For this review, take the finished solid that the model builds, in its own axes (mm). A direction names the side the tool comes from. Give positions to 0.01 mm unless a question says otherwise; leave off trailing zeros. Loops run counter-clockwise (first coordinate to the right, second up) from the corner with the lowest first, then second, coordinate; pieces in that order, holes last.
```python
from build123d import *

# Parameters (mm, degrees)
F0_W     = 20
F0_H     = 20
F1_DEPTH = 23
F2_W     = 20
F2_H     = 20
F3_DEPTH = 2
F3_TAPER = 30
F6_R     = 2


with BuildPart() as f1:
    # F0 (on Top) → F1 (new body)
    with BuildSketch(Plane.XY):
        Rectangle(F0_W, F0_H)
    extrude(amount=F1_DEPTH)

    # F2 (on face) → F3 (join)
    with BuildSketch(Plane.XY.offset(23)):
        Rectangle(F2_W, F2_H)
    extrude(amount=F3_DEPTH, taper=F3_TAPER)

    # F4 (on Front) → F5 (revolve)
    with BuildSketch(Plane.XZ):
        Polygon((0, -56), (0, 0), (-10, 0), (-7, -8), (-7, -50), (-5, -50), (-5, -56), align=None)
    revolve(axis=Axis((0, 0, -28), (0, 0, -1)))

    # F6
    f6_edges = [f1.edges().sort_by_distance(p)[0] for p in [
        (-10, 10, 11.5),
        (-10, -10, 11.5),
        (10, -10, 11.5),
        (10, 10, 11.5),
    ]]
    fillet(f6_edges, radius=F6_R)


solid = f1.part
```
Q1. For pin 1 Ø1 at (y, z) = (6, -42) entering from +X; pin 2 Ø11 at (x, y) = (-5.5, 7.5) entering from -Z; pin 3 Ø3 at (x, y) = (-4.5, -6.5) entering from -Z; pin 4 Ø1 at (x, z) = (-5.5, -46) entering from -Y, all flat-tipped, find the tip position at first contact; note any pin that passes through.
Answers:
pin 1: stops at x = 4.33
pin 2: stops at z = -56
pin 3: stops at z = -50
pin 4: stops at y = -4.9
Q2. For probe 1 along Z at (x, y) = (-2.75, -6); probe 2 along Z at (x, y) = (7.25, 7.25); probe 3 along X at (y, z) = (5.5, -10), list the stretches that pass through material, from the lowest coordinate up.
Answers:
probe 1: z = -50 to 25
probe 2: z = 0 to 25
probe 3: x = -4.33 to 4.33
Q3. Mouldability with a two-part tool opening along X and no side actions: class faces 1 (the cylindrical face through (-9.43, -9.4, 12.18)), 2 (the cylindrical face through (9.4, -9.43, 12.18)), 3 (the flat face through (2, 5, -50)) as +X half, -X half, draft (parallel to the pull), parting line (faces both ways), or undercut.
Answers:
face 1: -X half
face 2: +X half
face 3: draft
Q4. Consider section A-A on z = -15.5. Give the boundary of the cut face in (x, y), plus the area to 3 significant figures.
Answers:
outline: circle Ø14 at (0, 0)
area: 154 mm2
Q5. Machinability: for faces 4 (the flat face through (8, -8, 0)), 5 (the flat face through (8, 8, 0)), 6 (the flat face through (-8, 8, 0)), which of the approach directions +Z, -Z, +X, -X, +Y, -Y give a long, thin tool a straight path to every point of the face, cutting with its end or side? Answer none if there is none.
Answers:
face 4: -Z, +X, -Y
face 5: -Z, +X, +Y
face 6: -Z, -X, +Y
